Read the model definition and answer for the solid it produces. Units are mm, in the model's axes. A direction names the side the tool comes from. Coordinates: 2 decimals unless noted, no trailing zeros. Order: outer loops, then holes, each group sorted by start corner. A loop starts at its lowest first (then second) coordinate and runs counter-clockwise, first axis right, second up. Notation, with made-up numbers: (-5.5, 27) -> (34.5, 27) arc R16 ccw to (34.5, 53) -> close; hole circle Ø8 at (-26.75, 77.25). An arc over 180 degrees is marked (long way). Answer as a JSON object with one key per item and string values. Group by question number.
1) Determine the mould class of faces 4 (the flat face through (10, 10, -2)), 5 (the flat face through (10, 15, 0)), 6 (the flat face through (10, 22, -1)), 7 (the flat face through (10, 0, -5)) for opening direction Y: released by +Y, released by -Y, zero draft, split by the parting line, or undercut.
2) Section A-A on z = -1.25 is taken. Determine the outline of the cut face in (x, y), and give its area (3 significant figures).
3) A tool of negligible diameter and unlimited length cuts with its end or side. For faces 1 (the flat face through (10, 18, -1)), 2 (the cylindrical face through (5.604, 25.193, -7.473)), 3 (the flat face through (10, 2, 0)), from which of +Z, -Z, +X, -X, +Y, -Y can it reach the whole face along a straight path? Write none if from no direction.
4) Section D-D on z = -11.25 is taken. Determine the outline of the cut face in (x, y).
5) Section B-B on y = 25 is taken. Determine the outline of the cut face in (x, z), and give its area (3 significant figures).
6) Given pin 1 (4.5 mm diameter, centred on x = 10, y = 5, fed in from -Z); pin 2 (2 mm diameter, centred on x = 7.5, z = -0.5, fed in from -Y); pin 3 (5.5 mm diameter, centred on x = 10, y = 25, fed in from -Z); pin 4 (9.5 mm diameter, centred on x = 8, y = 26.5, fed in from -Z), each flat-ended and moving along its own axis, determine where each tip first touches the part or whether it passes through.
7) Consider L1, parallel to Y at x = 10, z = -6.75; L2, parallel to Y at x = 10, z = -3; L3, parallel to X at y = 25, z = -9. Determine where each line is inside the solid, lowest interval first.
8) Section C-C on x = 10 is taken. Determine the outline of the cut face in (y, z).
from build123d import *

# Parameters (mm, degrees)
BOSS_EXTRUDE1_DEPTH = 30
CUT_EXTRUDE1_REACH  = 15
SKETCH2_R           = 2.6
CUT_EXTRUDE2_REACH  = 19.5
CUT_EXTRUDE2_START  = -4.5
SKETCH3_R           = 4.4
CUT_EXTRUDE3_REACH  = 22
SKETCH4_W           = 2
SKETCH4_H           = 4


with BuildPart() as part:
    # Sketch1 → Boss-Extrude1 (new body)
    with BuildSketch(Plane(origin=(0, 0, 0), x_dir=(1, 0, 0), z_dir=(0, 1, 0))):
        with BuildLine():
            Line((0, 0), (20, 0))
            Line((20, 0), (20, 13))
            ThreePointArc((20, 13), (10, 9.966629547), (0, 13))
            Line((0, 13), (0, 0))
        make_face()
    extrude(amount=BOSS_EXTRUDE1_DEPTH)

    # Sketch2 → Cut-Extrude1 (cut, up to next)
    with BuildSketch(Plane.XY, mode=Mode.PRIVATE) as cut_extrude1_sk1:
        with Locations((10, 25)):
            Circle(SKETCH2_R)
    cut_extrude1_tool1 = extrude(cut_extrude1_sk1.sketch, amount=-CUT_EXTRUDE1_REACH, mode=Mode.PRIVATE) & part.part
    add(cut_extrude1_tool1.solids().sort_by_distance((10, 25, 0))[0], mode=Mode.SUBTRACT)
    # Sketch2 → Cut-Extrude1 (cut, up to next)
    with BuildSketch(Plane.XY, mode=Mode.PRIVATE) as cut_extrude1_sk2:
        with Locations((10, 5)):
            Circle(SKETCH2_R)
    cut_extrude1_tool2 = extrude(cut_extrude1_sk2.sketch, amount=-CUT_EXTRUDE1_REACH, mode=Mode.PRIVATE) & part.part
    add(cut_extrude1_tool2.solids().sort_by_distance((10, 5, 0))[0], mode=Mode.SUBTRACT)

    # Sketch3 → Cut-Extrude2 (cut, up to next)
    with BuildSketch(Plane.XY.offset(CUT_EXTRUDE2_START), mode=Mode.PRIVATE) as cut_extrude2_sk1:
        with Locations((10, 25)):
            Circle(SKETCH3_R)
    cut_extrude2_tool1 = extrude(cut_extrude2_sk1.sketch, amount=-CUT_EXTRUDE2_REACH, mode=Mode.PRIVATE) & part.part
    add(cut_extrude2_tool1.solids().sort_by_distance((10, 25, -4.5))[0], mode=Mode.SUBTRACT)
    # Sketch3 → Cut-Extrude2 (cut, up to next)
    with BuildSketch(Plane.XY.offset(CUT_EXTRUDE2_START), mode=Mode.PRIVATE) as cut_extrude2_sk2:
        with Locations((10, 5)):
            Circle(SKETCH3_R)
    cut_extrude2_tool2 = extrude(cut_extrude2_sk2.sketch, amount=-CUT_EXTRUDE2_REACH, mode=Mode.PRIVATE) & part.part
    add(cut_extrude2_tool2.solids().sort_by_distance((10, 5, -4.5))[0], mode=Mode.SUBTRACT)

    # Sketch4 → Cut-Extrude3 (cut, up to next)
    with BuildSketch(Plane(origin=(20, 0, 0), x_dir=(0, 0, -1), z_dir=(1, 0, 0)), mode=Mode.PRIVATE) as cut_extrude3_sk1:
        with Locations((1, 20)):
            Rectangle(SKETCH4_W, SKETCH4_H)
    cut_extrude3_tool1 = extrude(cut_extrude3_sk1.sketch, amount=-CUT_EXTRUDE3_REACH, mode=Mode.PRIVATE) & part.part
    add(cut_extrude3_tool1.solids().sort_by_distance((20, 20, -1))[0], mode=Mode.SUBTRACT)
    # Sketch4 → Cut-Extrude3 (cut, up to next)
    with BuildSketch(Plane(origin=(20, 0, 0), x_dir=(0, 0, -1), z_dir=(1, 0, 0)), mode=Mode.PRIVATE) as cut_extrude3_sk2:
        with Locations((1, 10)):
            Rectangle(SKETCH4_W, SKETCH4_H)
    cut_extrude3_tool2 = extrude(cut_extrude3_sk2.sketch, amount=-CUT_EXTRUDE3_REACH, mode=Mode.PRIVATE) & part.part
    add(cut_extrude3_tool2.solids().sort_by_distance((20, 10, -1))[0], mode=Mode.SUBTRACT)


solid = part.part
Worked answers:
{
 "1": {"face 4": "undercut", "face 5": "zero draft", "face 6": "undercut", "face 7": "released by -Y"},
 "2": {"outline": "(0, 0) -> (20, 0) -> (20, 8) -> (0, 8) -> close; (0, 12) -> (20, 12) -> (20, 18) -> (0, 18) -> close; (0, 22) -> (20, 22) -> (20, 30) -> (0, 30) -> close; hole circle Ø5.2 at (10, 5); hole circle Ø5.2 at (10, 25)", "area": "398 mm²"},
 "3": {"face 1": "+Z, +X, -X", "face 2": "-Z", "face 3": "+Z, +X, -X, +Y, -Y"},
 "4": {"outline": "(0, 0) -> (3.33, 0) -> (3.33, 30) -> (0, 30) -> close; (16.67, 0) -> (20, 0) -> (20, 30) -> (16.67, 30) -> close"},
 "5": {"outline": "(0, -13) arc R18 cw to (5.6, -10.51) -> (5.6, -4.5) -> (7.4, -4.5) -> (7.4, 0) -> (0, 0) -> close; (12.6, -4.5) -> (14.4, -4.5) -> (14.4, -10.51) arc R18 cw to (20, -13) -> (20, 0) -> (12.6, 0) -> close", "area": "146 mm²"},
 "6": {"pin 1": "passes through", "pin 2": "stops at y = 0", "pin 3": "stops at z = -4.5", "pin 4": "stops at z = -11.28"},
 "7": {"L1": "y = 0 to 0.6, 9.4 to 20.6, 29.4 to 30", "L2": "y = 0 to 2.4, 7.6 to 22.4, 27.6 to 30", "L3": "x = 0 to 5.6, 14.4 to 20"},
 "8": {"outline": "(0, -9.97) -> (0.6, -9.97) -> (0.6, -4.5) -> (2.4, -4.5) -> (2.4, 0) -> (0, 0) -> close; (7.6, -4.5) -> (9.4, -4.5) -> (9.4, -9.97) -> (20.6, -9.97) -> (20.6, -4.5) -> (22.4, -4.5) -> (22.4, 0) -> (22, 0) -> (22, -2) -> (18, -2) -> (18, 0) -> (12, 0) -> (12, -2) -> (8, -2) -> (8, 0) -> (7.6, 0) -> close; (27.6, -4.5) -> (29.4, -4.5) -> (29.4, -9.97) -> (30, -9.97) -> (30, 0) -> (27.6, 0) -> close"}
}
